The model under review builds one solid part; all positions refer to its coordinate system, in mm. Face numbers are marked on the shaded views. A direction names the side the tool comes from. Round coordinates to 2 decimals unless told otherwise and drop trailing zeros. Write each loop counter-clockwise with the first axis right and the second up, starting at its lowest first coordinate (ties: lowest second). Pieces come first, ordered by that corner, then holes. Notation, with made-up numbers: (25, 35) - (35, 35) arc R7 ccw to (35, 44) - close; hole circle Ø3 at (36.25, 6.25). An arc over 180 degrees is marked (long way). Write each question's results on one line, items separated by ' | '.
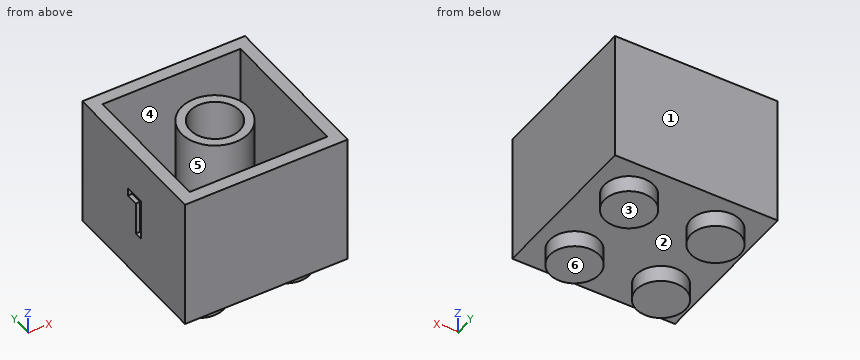
```python
from build123d import *

# Parameters (mm, degrees)
SKETCH2_W           = 15.8
SKETCH2_H           = 15.8
BOSS_EXTRUDE1_DEPTH = 12.7
CUT_EXTRUDE1_DEPTH  = 11.49999986
SKETCH5_R           = 3.256854249
BOSS_EXTRUDE3_DEPTH = 11.5
SKETCH6_R           = 2.4
CUT_EXTRUDE2_DEPTH  = 11.5
SKETCH4_R           = 2.4
BOSS_EXTRUDE4_DEPTH = 1.6
SKETCH7_R           = 1.2
CUT_EXTRUDE3_DEPTH  = 1.6
CUT_EXTRUDE4_DEPTH  = 0.4


with BuildPart() as part:
    # Sketch2 → Boss-Extrude1 (new body)
    with BuildSketch(Plane(origin=(0, 0, 0), x_dir=(0, 1, 0), z_dir=(0, 0, 1))):
        Rectangle(SKETCH2_W, SKETCH2_H)
    extrude(amount=BOSS_EXTRUDE1_DEPTH)

    # 3DSketch1 → Cut-Extrude1 (cut)
    with BuildSketch(Plane(origin=(-6.7, -6.7, 12.7), x_dir=(0.7071067811865477, 0.7071067811865474, 0), z_dir=(0, 0, 1))):
        Polygon((0, 0), (9.475230868, -9.475230868), (18.950461736, 0), (9.475230868, 9.475230868), align=None)
    extrude(amount=-CUT_EXTRUDE1_DEPTH, mode=Mode.SUBTRACT)

    # Sketch5 → Boss-Extrude3 (add)
    with BuildSketch(Plane.XY.offset(1.20000014)):
        with Locations(Location((0, 0, 0), (0, 0, 180))):
            Circle(SKETCH5_R)
    extrude(amount=BOSS_EXTRUDE3_DEPTH)

    # Sketch6 → Cut-Extrude2 (cut)
    with BuildSketch(Plane.XY.offset(12.70000014)):
        Circle(SKETCH6_R)
    extrude(amount=-CUT_EXTRUDE2_DEPTH, mode=Mode.SUBTRACT)

    # Sketch4 → Boss-Extrude4 (add)
    with BuildSketch(Plane(origin=(0, 0, 0), x_dir=(1, 0, 0), z_dir=(0, 0, -1))):
        with Locations(Location((-4.2, 4.2, 0), (0, 0, 180))):
            Circle(SKETCH4_R)
        with Locations(Location((4.2, 4.2, 0), (0, 0, 180))):
            Circle(SKETCH4_R)
        with Locations(Location((-4.2, -4.2, 0), (0, 0, 180))):
            Circle(SKETCH4_R)
        with Locations(Location((4.2, -4.2, 0), (0, 0, 180))):
            Circle(SKETCH4_R)
    extrude(amount=BOSS_EXTRUDE4_DEPTH)

    # Sketch7 → Cut-Extrude3 (cut)
    with BuildSketch(Plane.XY.offset(1.20000014)):
        with Locations((-4.3, 4.3)):
            Circle(SKETCH7_R)
        with Locations(Location((4.3, 4.3, 0), (0, 0, 180))):
            Circle(SKETCH7_R)
        with Locations((4.3, -4.3)):
            Circle(SKETCH7_R)
        with Locations(Location((-4.3, -4.3, 0), (0, 0, 180))):
            Circle(SKETCH7_R)
    extrude(amount=-CUT_EXTRUDE3_DEPTH, mode=Mode.SUBTRACT)

    # Sketch8 → Cut-Extrude4 (cut)
    with BuildSketch(Plane(origin=(-7.9, 0, 0), x_dir=(0, -1, 0), z_dir=(-1, 0, 0))):
        Polygon((0.322443159, 4.35), (0.322443159, 7.55), (-0.877556841, 7.55), (-0.877556841, 8.35), (1.122443159, 8.35), (1.122443159, 4.35), align=None)
    extrude(amount=-CUT_EXTRUDE4_DEPTH, mode=Mode.SUBTRACT)


solid = part.part
```
Q1. For probe 1 along Y at (x, z) = (0, 6.5); probe 2 along Y at (x, z) = (4.3, 0.8); probe 3 along X at (y, z) = (3, 12), list the stretches that pass through material, from the lowest coordinate up.
Evaluation:
probe 1: y = -7.9 to -6.7, -3.26 to -2.4, 2.4 to 3.26, 6.7 to 7.9 | probe 2: y = -7.9 to -5.5, -3.1 to 3.1, 5.5 to 7.9 | probe 3: x = -7.9 to -6.7, -1.27 to 1.27, 6.7 to 7.9
Q2. Tool access review of the marked faces 5 and 6: name each direction out of +Z, -Z, +X, -X, +Y, -Y from which nothing blocks a thin tool from reaching the whole face with its end or side.
Evaluation:
face 5: +Z | face 6: -Z, +X, -X, +Y, -Y
Q3. We need section A-A (z = 6.25). State the section outline as (x, y) points.
Evaluation:
outline: (-7.9, -7.9) - (7.9, -7.9) - (7.9, 7.9) - (-7.9, 7.9) - (-7.9, -0.32) - (-7.5, -0.32) - (-7.5, -1.12) - (-7.9, -1.12) - close; circle Ø6.51 at (0, 0); hole (-6.7, -6.7) - (6.7, -6.7) - (6.7, 6.7) - (-6.7, 6.7) - close; hole circle Ø4.8 at (0, 0)
Q4. The part is to be moulded in two halves that separate along Y. For the marked faces 1, 2, 3 and 4, say which applies: released by +Y, released by -Y, zero draft, split by the parting line, or undercut.
Evaluation:
face 1: released by +Y | face 2: undercut | face 3: zero draft | face 4: undercut
Q5. We need section C-C (y = 0). State the section outline as (x, z) points, plus the area to 3 significant figures.
Evaluation:
outline: (-7.9, 0) - (7.9, 0) - (7.9, 12.7) - (6.7, 12.7) - (6.7, 1.2) - (3.26, 1.2) - (3.26, 12.7) - (2.4, 12.7) - (2.4, 1.2) - (-2.4, 1.2) - (-2.4, 12.7) - (-3.26, 12.7) - (-3.26, 1.2) - (-6.7, 1.2) - (-6.7, 12.7) - (-7.9, 12.7) - (-7.9, 8.35) - (-7.5, 8.35) - (-7.5, 7.55) - (-7.9, 7.55) - close | area: 65.9 mm^2
Q6. Insertion check: P1, Ø4, axis at x = 0, y = 0, coming from the +Z side; P2, Ø1.4, axis at x = -4.3, y = -4.3, coming from the +Z side. Each pin has a flat end and moves straight along its axis. Give the tip position at first contact, or say it passes through.
Evaluation:
P1: stops at z = 1.2 | P2: stops at z = -0.4
Q7. We need section D-D (z = 4). State the section outline as (x, y) points.
Evaluation:
outline: (-7.9, -7.9) - (7.9, -7.9) - (7.9, 7.9) - (-7.9, 7.9) - close; circle Ø6.51 at (0, 0); hole (-6.7, -6.7) - (6.7, -6.7) - (6.7, 6.7) - (-6.7, 6.7) - close; hole circle Ø4.8 at (0, 0)
Q8. We need section B-B (x = 0). State the section outline as (y, z) points.
Evaluation:
outline: (-7.9, 0) - (7.9, 0) - (7.9, 12.7) - (6.7, 12.7) - (6.7, 1.2) - (3.26, 1.2) - (3.26, 12.7) - (2.4, 12.7) - (2.4, 1.2) - (-2.4, 1.2) - (-2.4, 12.7) - (-3.26, 12.7) - (-3.26, 1.2) - (-6.7, 1.2) - (-6.7, 12.7) - (-7.9, 12.7) - close
